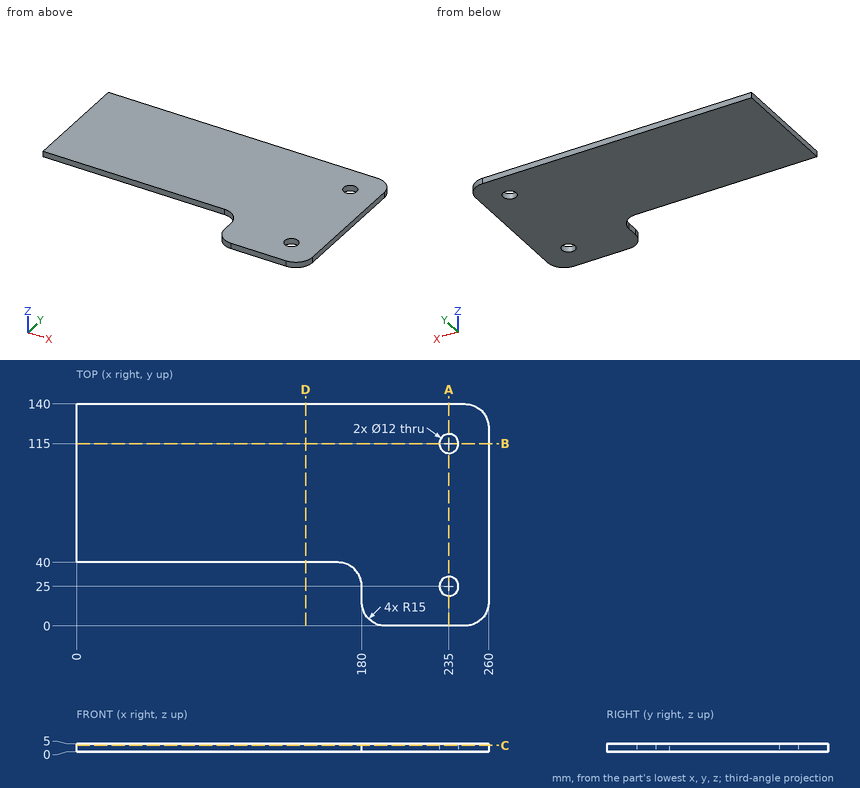
Could you check a few things on this drawing? It's one solid part, dimensions in mm from its lowest x, y, z. Coordinates: 2 decimals unless noted, no trailing zeros. Order: outer loops, then holes, each group sorted by start corner. A loop starts at its lowest first (then second) coordinate and runs counter-clockwise, first axis right, second up.
1. If we section it at A-A (x = 235): Please give me the cut outline in (y, z), then the cut area to 3 significant figures.
2. I'm going to push a flat-ended pin straight in: pin 1 (3 mm diameter, centred on x = 181.5, z = 1.5, fed in from -Y). Where does the tip first touch, or does it pass through?
3. I need wall thicknesses on line 1 (Y direction, x = 235, z = 1.1); line 2 (Y direction, x = 239, z = 3.25); line 3 (X direction, y = 25, z = 1.4). Which ranges of each line are inside material? Lowest first, please.
4. If we section it at B-B (y = 115): Please give me the cut outline in (x, z).
5. If we section it at D-D (x = 144.5): Please give me the cut outline in (y, z), then the cut area to 3 significant figures.
6. If we section it at C-C (z = 4): Please give me the cut outline in (x, y).
Entries:
1. outline: (0, 0) - (19, 0) - (19, 5) - (0, 5) - close; (31, 0) - (109, 0) - (109, 5) - (31, 5) - close; (121, 0) - (140, 0) - (140, 5) - (121, 5) - close
1. area: 580 mm2
2. pin 1: stops at y = 6
3. line 1: y = 0 to 19, 31 to 109, 121 to 140
3. line 2: y = 0 to 20.53, 29.47 to 110.53, 119.47 to 140
3. line 3: x = 180 to 229, 241 to 260
4. outline: (0, 0) - (229, 0) - (229, 5) - (0, 5) - close; (241, 0) - (260, 0) - (260, 5) - (241, 5) - close
5. outline: (40, 0) - (140, 0) - (140, 5) - (40, 5) - close
5. area: 500 mm2
6. outline: (0, 40) - (165, 40) arc R15 cw to (180, 25) - (180, 15) arc R15 ccw to (195, 0) - (245, 0) arc R15 ccw to (260, 15) - (260, 125) arc R15 ccw to (245, 140) - (0, 140) - close; hole circle Ø12 at (235, 25); hole circle Ø12 at (235, 115)
